Here's how the part is built. I have some questions about the finished solid (model axes, mm). Face numbers are marked on the shaded views. A direction names the side the tool comes from. Round coordinates to 2 decimals unless told otherwise and drop trailing zeros. Order: outer loops, then holes, each group sorted by start corner. A loop starts at its lowest first (then second) coordinate and runs counter-clockwise, first axis right, second up. Notation, with made-up numbers: (20.25, -26) -> (30.25, -26) arc R13 ccw to (30.25, -13) -> close; hole circle Ø3 at (74, -17.5). An arc over 180 degrees is marked (long way). Use a Markdown table: item, result. Add a question column.
(1) I'm going to push flat-ended pins straight in: P1, Ø6, axis at x = 42.5, y = 58, coming from the -Z side; P2, Ø6, axis at y = 84.5, z = 13.5, coming from the +X side; P3, Ø3, axis at y = 67.5, z = 112, coming from the -X side. Where does each tip first touch, or does it pass through?
(2) I want a section at A-A, the plane y = 58.5. Please give me the cut outline in (x, z), then the cut area to 3 significant figures.
(3) I want a section at C-C, the plane x = 197. Please give me the cut outline in (y, z).
(4) Thinking about a two-plate mould opening in X: for the marked faces 3, 4 and 5, which applies, pulls with the +X half, pulls with the -X half, needs draft (parallel to the pull), parting line crosses it, or undercut?
(5) If I drill on probe 1 along Z at (x, y) = (203, 16); probe 2 along X at (y, z) = (12, 28); probe 3 along X at (y, z) = (57, 7.5), over which ranges is the centre line in solid material (lowest first)?
(6) I want a section at B-B, the plane z = 129. Please give me the cut outline in (x, y), then the cut area to 3 significant figures.
(7) On a 3-axis mill with a long thin cutter (end or side, diameter ignored), from which of +Z, -Z, +X, -X, +Y, -Y can I reach the whole of each face in a straight line? I mean the marked faces 1 and 2. Say none if no direction works.
(8) I want a section at D-D, the plane z = 23.5. Please give me the cut outline in (x, y), then the cut area to 3 significant figures.
from build123d import *

# Parameters (mm, degrees)
F1_DEPTH = 100


with BuildPart() as f1:
    # F0 (on Front) → F1 (new body)
    with BuildSketch(Plane.XZ):
        with BuildLine():
            ThreePointArc((-146.068349, 5.22981), (14.418385, 145.138901), (174.905118, 5.22981))
            ThreePointArc((174.905118, 5.22981), (179.57454, -3.413996), (188.774342, -6.861099))
            Line((188.774342, -6.861099), (231.418385, -6.861099))
            Line((231.418385, -6.861099), (231.418385, -0.861099))
            Line((231.418385, -0.861099), (188.774342, -0.861099))
            ThreePointArc((188.774342, -0.861099), (183.517312, 1.108674), (180.849072, 6.047992))
            ThreePointArc((180.849072, 6.047992), (14.418385, 151.138901), (-152.012302, 6.047992))
            ThreePointArc((-152.012302, 6.047992), (-154.680543, 1.108674), (-159.937573, -0.861099))
            Line((-159.937573, -0.861099), (-202.581615, -0.861099))
            Line((-202.581615, -0.861099), (-202.581615, -6.861099))
            Line((-202.581615, -6.861099), (-159.937573, -6.861099))
            ThreePointArc((-159.937573, -6.861099), (-150.737771, -3.413996), (-146.068349, 5.22981))
        make_face()
    extrude(amount=-F1_DEPTH)


solid = f1.part
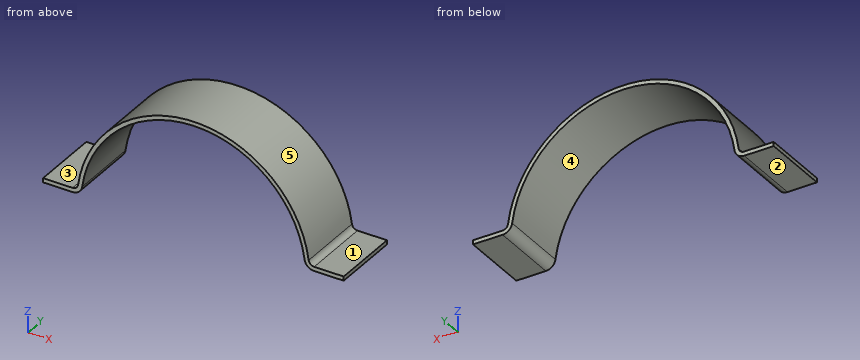
Taken from the geometry:
| question | item | result |
|---|---|---|
| 1 | P1 | stops at z = 142.13 |
| 1 | P2 | stops at x = 180.18 |
| 1 | P3 | stops at x = -95.14 |
| 2 | outline | (-202.58, -6.86) -> (-159.94, -6.86) arc R14 ccw to (-146.07, 5.23) arc R162 cw to (174.91, 5.23) arc R14 ccw to (188.77, -6.86) -> (231.42, -6.86) -> (231.42, -0.86) -> (188.77, -0.86) arc R8 cw to (180.85, 6.05) arc R168 ccw to (-152.01, 6.05) arc R8 cw to (-159.94, -0.86) -> (-202.58, -0.86) -> close |
| 2 | area | 3,540 mm2 |
| 3 | outline | (0, -6.86) -> (100, -6.86) -> (100, -0.86) -> (0, -0.86) -> close |
| 4 | face 3 | needs draft |
| 4 | face 4 | undercut |
| 4 | face 5 | parting line crosses it |
| 5 | probe 1 | z = -6.86 to -0.86 |
| 5 | probe 2 | x = -147.48 to -141.25, 170.08 to 176.32 |
| 5 | probe 3 | x = -151.81 to -145.74, 174.58 to 180.64 |
| 6 | outline | (-68.94, 0) -> (-56.07, 0) -> (-56.07, 100) -> (-68.94, 100) -> close; (84.91, 0) -> (97.78, 0) -> (97.78, 100) -> (84.91, 100) -> close |
| 6 | area | 2,570 mm2 |
| 7 | face 1 | +Z, +X, +Y, -Y |
| 7 | face 2 | -Z, +X, -X, +Y, -Y |
| 8 | outline | (-148.66, 0) -> (-142.47, 0) -> (-142.47, 100) -> (-148.66, 100) -> close; (171.31, 0) -> (177.5, 0) -> (177.5, 100) -> (171.31, 100) -> close |
| 8 | area | 1,240 mm2 |
